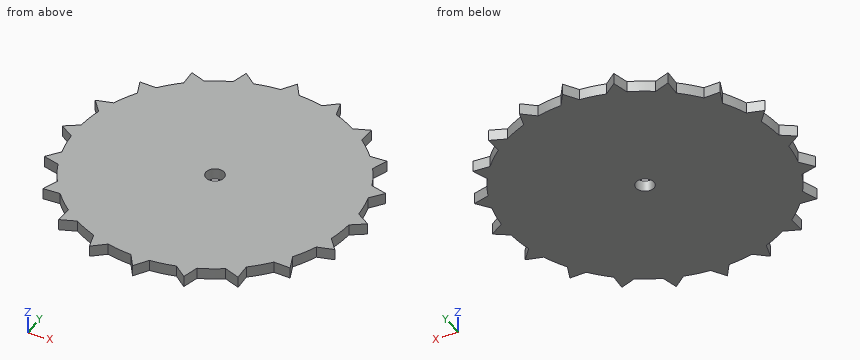
from build123d import *

# Parameters (mm, degrees)
F1_DEPTH = 3
F2_R     = 2.45
F3_DEPTH = 3


with BuildPart() as f1:
    # F0 (on Top) → F1 (new body)
    with BuildSketch(Plane.XY):
        with BuildLine():
            ThreePointArc((37.418773, -2.466863), (37.479688, -1.2341), (37.5, 0))
            ThreePointArc((37.5, 0), (37.479688, 1.2341), (37.418773, 2.466863))
            ThreePointArc((37.418773, 2.466863), (37.038313, 5.866292), (36.349671, 9.21691))
            ThreePointArc((36.349671, 9.21691), (35.664619, 11.588137), (34.825065, 13.909163))
            ThreePointArc((34.825065, 13.909163), (33.412745, 17.024644), (31.722409, 19.998469))
            ThreePointArc((31.722409, 19.998469), (30.338137, 22.041947), (28.822438, 23.989937))
            ThreePointArc((28.822438, 23.989937), (26.516504, 26.516504), (23.989937, 28.822438))
            ThreePointArc((23.989937, 28.822438), (22.041947, 30.338137), (19.998469, 31.722409))
            ThreePointArc((19.998469, 31.722409), (17.024644, 33.412745), (13.909163, 34.825065))
            ThreePointArc((13.909163, 34.825065), (11.588137, 35.664619), (9.21691, 36.349671))
            ThreePointArc((9.21691, 36.349671), (5.866292, 37.038313), (2.466863, 37.418773))
            ThreePointArc((2.466863, 37.418773), (0, 37.5), (-2.466863, 37.418773))
            ThreePointArc((-2.466863, 37.418773), (-5.866292, 37.038313), (-9.21691, 36.349671))
            ThreePointArc((-9.21691, 36.349671), (-11.588137, 35.664619), (-13.909163, 34.825065))
            ThreePointArc((-13.909163, 34.825065), (-17.024644, 33.412745), (-19.998469, 31.722409))
            ThreePointArc((-19.998469, 31.722409), (-22.041947, 30.338137), (-23.989937, 28.822438))
            ThreePointArc((-23.989937, 28.822438), (-26.516504, 26.516504), (-28.822438, 23.989937))
            ThreePointArc((-28.822438, 23.989937), (-30.338137, 22.041947), (-31.722409, 19.998469))
            ThreePointArc((-31.722409, 19.998469), (-33.412745, 17.024644), (-34.825065, 13.909163))
            ThreePointArc((-34.825065, 13.909163), (-35.664619, 11.588137), (-36.349671, 9.21691))
            ThreePointArc((-36.349671, 9.21691), (-37.038313, 5.866292), (-37.418773, 2.466863))
            ThreePointArc((-37.418773, 2.466863), (-37.5, 0), (-37.418773, -2.466863))
            ThreePointArc((-37.418773, -2.466863), (-37.038313, -5.866292), (-36.349671, -9.21691))
            ThreePointArc((-36.349671, -9.21691), (-35.664619, -11.588137), (-34.825065, -13.909163))
            ThreePointArc((-34.825065, -13.909163), (-33.412745, -17.024644), (-31.722409, -19.998469))
            ThreePointArc((-31.722409, -19.998469), (-30.338137, -22.041947), (-28.822438, -23.989937))
            ThreePointArc((-28.822438, -23.989937), (-26.516504, -26.516504), (-23.989937, -28.822438))
            ThreePointArc((-23.989937, -28.822438), (-22.041947, -30.338137), (-19.998469, -31.722409))
            ThreePointArc((-19.998469, -31.722409), (-17.024644, -33.412745), (-13.909163, -34.825065))
            ThreePointArc((-13.909163, -34.825065), (-11.588137, -35.664619), (-9.21691, -36.349671))
            ThreePointArc((-9.21691, -36.349671), (-5.866292, -37.038313), (-2.466863, -37.418773))
            ThreePointArc((-2.466863, -37.418773), (0, -37.5), (2.466863, -37.418773))
            ThreePointArc((2.466863, -37.418773), (5.866292, -37.038313), (9.21691, -36.349671))
            ThreePointArc((9.21691, -36.349671), (11.588137, -35.664619), (13.909163, -34.825065))
            ThreePointArc((13.909163, -34.825065), (17.024644, -33.412745), (19.998469, -31.722409))
            ThreePointArc((19.998469, -31.722409), (22.041947, -30.338137), (23.989937, -28.822438))
            ThreePointArc((23.989937, -28.822438), (26.516504, -26.516504), (28.822438, -23.989937))
            ThreePointArc((28.822438, -23.989937), (30.338137, -22.041947), (31.722409, -19.998469))
            ThreePointArc((31.722409, -19.998469), (33.412745, -17.024644), (34.825065, -13.909163))
            ThreePointArc((34.825065, -13.909163), (35.664619, -11.588137), (36.349671, -9.21691))
            ThreePointArc((36.349671, -9.21691), (37.038313, -5.866292), (37.418773, -2.466863))
        make_face()
        with BuildLine():
            ThreePointArc((37.418773, 2.466863), (37.479688, 1.2341), (37.5, 0))
            ThreePointArc((37.5, 0), (37.479688, -1.2341), (37.418773, -2.466863))
            Line((37.418773, -2.466863), (41.188397, 0))
            Line((41.188397, 0), (37.418773, 2.466863))
        make_face()
        with BuildLine():
            ThreePointArc((34.825065, 13.909163), (35.664619, 11.588137), (36.349671, 9.21691))
            Line((36.349671, 9.21691), (39.172493, 12.727915))
            Line((39.172493, 12.727915), (34.825065, 13.909163))
        make_face()
        with BuildLine():
            Line((39.172493, -12.727915), (36.349671, -9.21691))
            ThreePointArc((36.349671, -9.21691), (35.664619, -11.588137), (34.825065, -13.909163))
            Line((34.825065, -13.909163), (39.172493, -12.727915))
        make_face()
        with BuildLine():
            ThreePointArc((28.822438, 23.989937), (30.338137, 22.041947), (31.722409, 19.998469))
            Line((31.722409, 19.998469), (33.322113, 24.209932))
            Line((33.322113, 24.209932), (28.822438, 23.989937))
        make_face()
        with BuildLine():
            Line((33.322113, -24.209932), (31.722409, -19.998469))
            ThreePointArc((31.722409, -19.998469), (30.338137, -22.041947), (28.822438, -23.989937))
            Line((28.822438, -23.989937), (33.322113, -24.209932))
        make_face()
        with BuildLine():
            ThreePointArc((19.998469, 31.722409), (22.041947, 30.338137), (23.989937, 28.822438))
            Line((23.989937, 28.822438), (24.209932, 33.322113))
            Line((24.209932, 33.322113), (19.998469, 31.722409))
        make_face()
        with BuildLine():
            Line((24.209932, -33.322113), (23.989937, -28.822438))
            ThreePointArc((23.989937, -28.822438), (22.041947, -30.338137), (19.998469, -31.722409))
            Line((19.998469, -31.722409), (24.209932, -33.322113))
        make_face()
        with BuildLine():
            ThreePointArc((9.21691, 36.349671), (11.588137, 35.664619), (13.909163, 34.825065))
            Line((13.909163, 34.825065), (12.727915, 39.172493))
            Line((12.727915, 39.172493), (9.21691, 36.349671))
        make_face()
        with BuildLine():
            Line((12.727915, -39.172493), (13.909163, -34.825065))
            ThreePointArc((13.909163, -34.825065), (11.588137, -35.664619), (9.21691, -36.349671))
            Line((9.21691, -36.349671), (12.727915, -39.172493))
        make_face()
        with BuildLine():
            ThreePointArc((-2.466863, 37.418773), (0, 37.5), (2.466863, 37.418773))
            Line((2.466863, 37.418773), (0, 41.188397))
            Line((0, 41.188397), (-2.466863, 37.418773))
        make_face()
        with BuildLine():
            Line((0, -41.188397), (2.466863, -37.418773))
            ThreePointArc((2.466863, -37.418773), (0, -37.5), (-2.466863, -37.418773))
            Line((-2.466863, -37.418773), (0, -41.188397))
        make_face()
        with BuildLine():
            ThreePointArc((-13.909163, 34.825065), (-11.588137, 35.664619), (-9.21691, 36.349671))
            Line((-9.21691, 36.349671), (-12.727915, 39.172493))
            Line((-12.727915, 39.172493), (-13.909163, 34.825065))
        make_face()
        with BuildLine():
            Line((-12.727915, -39.172493), (-9.21691, -36.349671))
            ThreePointArc((-9.21691, -36.349671), (-11.588137, -35.664619), (-13.909163, -34.825065))
            Line((-13.909163, -34.825065), (-12.727915, -39.172493))
        make_face()
        with BuildLine():
            ThreePointArc((-23.989937, 28.822438), (-22.041947, 30.338137), (-19.998469, 31.722409))
            Line((-19.998469, 31.722409), (-24.209932, 33.322113))
            Line((-24.209932, 33.322113), (-23.989937, 28.822438))
        make_face()
        with BuildLine():
            Line((-24.209932, -33.322113), (-19.998469, -31.722409))
            ThreePointArc((-19.998469, -31.722409), (-22.041947, -30.338137), (-23.989937, -28.822438))
            Line((-23.989937, -28.822438), (-24.209932, -33.322113))
        make_face()
        with BuildLine():
            ThreePointArc((-31.722409, 19.998469), (-30.338137, 22.041947), (-28.822438, 23.989937))
            Line((-28.822438, 23.989937), (-33.322113, 24.209932))
            Line((-33.322113, 24.209932), (-31.722409, 19.998469))
        make_face()
        with BuildLine():
            Line((-33.322113, -24.209932), (-28.822438, -23.989937))
            ThreePointArc((-28.822438, -23.989937), (-30.338137, -22.041947), (-31.722409, -19.998469))
            Line((-31.722409, -19.998469), (-33.322113, -24.209932))
        make_face()
        with BuildLine():
            ThreePointArc((-36.349671, 9.21691), (-35.664619, 11.588137), (-34.825065, 13.909163))
            Line((-34.825065, 13.909163), (-39.172493, 12.727915))
            Line((-39.172493, 12.727915), (-36.349671, 9.21691))
        make_face()
        with BuildLine():
            Line((-39.172493, -12.727915), (-34.825065, -13.909163))
            ThreePointArc((-34.825065, -13.909163), (-35.664619, -11.588137), (-36.349671, -9.21691))
            Line((-36.349671, -9.21691), (-39.172493, -12.727915))
        make_face()
        with BuildLine():
            ThreePointArc((-37.418773, -2.466863), (-37.5, 0), (-37.418773, 2.466863))
            Line((-37.418773, 2.466863), (-41.188397, 0))
            Line((-41.188397, 0), (-37.418773, -2.466863))
        make_face()
    extrude(amount=F1_DEPTH)

    # F2 (on face) → F3 (cut)
    with BuildSketch(Plane.XY.offset(3)):
        Circle(F2_R)
    extrude(amount=-F3_DEPTH, mode=Mode.SUBTRACT)


solid = f1.part
Verification items for the finished model (mm, model axes). Coordinates: 2 decimals unless noted, no trailing zeros. Write each loop counter-clockwise with the first axis right and the second up, starting at its lowest first coordinate (ties: lowest second). Pieces come first, ordered by that corner, then holes. Notation, with made-up numbers: (20, -30) -> (53, -30) arc R6 ccw to (53, -23) -> close; hole circle Ø1 at (30, 19.25). An arc over 180 degrees is marked (long way). One line per item, written item: value. Start each with the question number.
Q1. Cross-section at C-C on y = 6. Enter the section's corners in (x, z).
Q2. Go/stop test with flat-tipped pins: P1, Ø6, axis at x = 28.5, y = 32, coming from the +Z side; P2, Ø1.5, axis at y = -30, z = 2.5, coming from the +X side. Record where each tip stops, or that it passes through.
Q3. Cross-section at B-B on y = 21. Enter the section's corners in (x, z), and give its area (3 significant figures).
Q4. Thickness scan on L1, parallel to Y at x = -31.5, z = 2.8; L2, parallel to Y at x = 10, z = 1.3; L3, parallel to X at y = -10.5, z = 2.7. Record the ranges inside material, lowest first. Write a range as from..to.
Q5. Cross-section at A-A on x = -1. Enter the section's corners in (y, z).
Checked values:
1. outline: (-37.02, 0) -> (37.02, 0) -> (37.02, 3) -> (-37.02, 3) -> close
2. P1: passes through
2. P2: stops at x = 24.08
3. outline: (-32.1, 0) -> (32.1, 0) -> (32.1, 3) -> (-32.1, 3) -> close
3. area: 193 mm²
4. L1: y = -24.12..24.12
4. L2: y = -36.98..36.98
4. L3: x = -37.38..37.38
5. outline: (-39.66, 0) -> (-2.24, 0) -> (-2.24, 3) -> (-39.66, 3) -> close; (2.24, 0) -> (39.66, 0) -> (39.66, 3) -> (2.24, 3) -> close
